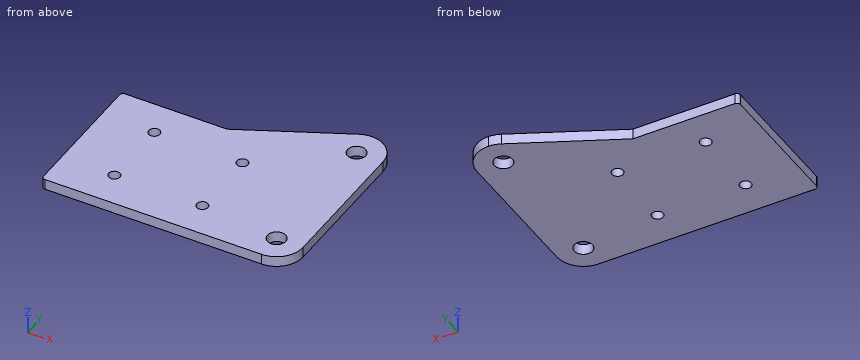
from build123d import *

# Parameters (mm, degrees)
SKETCH_1_R          = 2.6
EXTRUDE_1_DEPTH     = 3
CUT_EXTRUDE_START   = -3
CUT_EXTRUDE_1_DEPTH = 3
SKETCH_3_R          = 1.6
CUT_EXTRUDE_2_DEPTH = 3
FILLET_1_R          = 1


with BuildPart() as part:
    # 草图1 → 凸台-拉伸1 (new body)
    with BuildSketch(Plane.XY):
        with BuildLine():
            Line((-35, -27.5), (27.5, -27.5))
            ThreePointArc((27.5, -27.5), (32.803300859, -25.303300859), (35, -20))
            Line((35, -20), (35, 20))
            ThreePointArc((35, 20), (32.803300859, 25.303300859), (27.5, 27.5))
            Line((27.5, 27.5), (-35, 27.5))
            Line((-35, 27.5), (-35, -27.5))
        make_face()
        with Locations((27.5, 20)):
            Circle(SKETCH_1_R, mode=Mode.SUBTRACT)
        with Locations(Location((27.5, -20, 0), (0, 0, 180))):
            Circle(SKETCH_1_R, mode=Mode.SUBTRACT)
    extrude(amount=EXTRUDE_1_DEPTH)

    # 草图2 → 切除-拉伸1 (cut)
    with BuildSketch(Plane.XY.offset(3).offset(CUT_EXTRUDE_START)):
        with BuildLine():
            Line((-35, 12.5), (-5, 12.5))
            Line((-5, 12.5), (24.213483146, 26.741573034))
            ThreePointArc((24.213483146, 26.741573034), (25.8135537, 27.307933968), (27.5, 27.5))
            Line((27.5, 27.5), (27.5, 37.5))
            Line((27.5, 37.5), (-35, 37.5))
            Line((-35, 37.5), (-35, 12.5))
        make_face()
    extrude(amount=CUT_EXTRUDE_1_DEPTH, mode=Mode.SUBTRACT)

    # 草图3 → 切除-拉伸2 (cut)
    with BuildSketch(Plane.XY.offset(3)):
        with Locations((-20, 2.5)):
            Circle(SKETCH_3_R)
        with Locations(Location((5, 2.5, 0), (0, 0, 180))):
            Circle(SKETCH_3_R)
        with Locations((5, -17.5)):
            Circle(SKETCH_3_R)
        with Locations(Location((-20, -17.5, 0), (0, 0, 180))):
            Circle(SKETCH_3_R)
    extrude(amount=-CUT_EXTRUDE_2_DEPTH, mode=Mode.SUBTRACT)

    # 圆角1
    fillet_1_edges = [part.edges().sort_by_distance(p)[0] for p in [
        (-35, -27.5, 1.5),
        (-35, 12.5, 1.5),
    ]]
    fillet(fillet_1_edges, radius=FILLET_1_R)


solid = part.part
Source: CAD feature listing. Evaluate the final solid. Frame: model axes, mm. Coordinates: 2 decimals unless noted, no trailing zeros. Order: outer loops, then holes, each group sorted by start corner. A loop starts at its lowest first (then second) coordinate and runs counter-clockwise, first axis right, second up. Notation, with made-up numbers: M 7,15 L 51,15 A26 ccw 51,39 Z; hole C 85.25,2.5 d1. An arc over 180 degrees is marked long. Write each question's results on one line, items separated by ' | '. Start each with the question number.
Item 1: Line query: probe 1 along Y at (x, z) = (-20, 2.3); probe 2 along Y at (x, z) = (27.5, 2.35); probe 3 along Y at (x, z) = (-8, 2.35). Output: solid intervals per line, ascending.
Item 2: Cut plane D-D (x = -29). Return loops of the section in (y, z).
Item 3: Cut plane B-B (z = 2). Return loops of the section in (x, y).
Item 4: Cut plane C-C (y = 2.5). Return loops of the section in (x, z).
Item 5: Cut plane A-A (x = -20). Return loops of the section in (y, z), and give its area (3 significant figures).
Item 6: First-contact query: pin 1 Ø1 at (y, z) = (-21, 0.5) entering from +X; pin 2 Ø1.5 at (y, z) = (17.5, 2) entering from -X; pin 3 Ø1.5 at (x, z) = (-26.5, 2) entering from +Y. Flat tips, straight axial feed; report the tip coordinate or a pass-through.
Checked values:
1) probe 1: y = -27.5 to -19.1, -15.9 to 0.9, 4.1 to 12.5 | probe 2: y = -27.5 to -22.6, -17.4 to 17.4, 22.6 to 27.5 | probe 3: y = -27.5 to 12.5
2) outline: M -27.5,0 L 12.5,0 L 12.5,3 L -27.5,3 Z
3) outline: M -35,-26.5 A1 ccw -34,-27.5 L 27.5,-27.5 A7.5 ccw 35,-20 L 35,20 A7.5 ccw 24.21,26.74 L -5,12.5 L -34,12.5 A1 ccw -35,11.5 Z; hole C -20,-17.5 d3.2; hole C -20,2.5 d3.2; hole C 5,-17.5 d3.2; hole C 5,2.5 d3.2; hole C 27.5,-20 d5.2; hole C 27.5,20 d5.2
4) outline: M -35,0 L -21.6,0 L -21.6,3 L -35,3 Z; M -18.4,0 L 3.4,0 L 3.4,3 L -18.4,3 Z; M 6.6,0 L 35,0 L 35,3 L 6.6,3 Z
5) outline: M -27.5,0 L -19.1,0 L -19.1,3 L -27.5,3 Z; M -15.9,0 L 0.9,0 L 0.9,3 L -15.9,3 Z; M 4.1,0 L 12.5,0 L 12.5,3 L 4.1,3 Z | area: 101 mm2
6) pin 1: stops at x = 34.98 | pin 2: stops at x = 3.72 | pin 3: stops at y = 12.5
